The model under review builds one solid part; all positions refer to its coordinate system, in mm. A direction names the side the tool comes from. Coordinates: 2 decimals unless noted, no trailing zeros. Loops run counter-clockwise (first coordinate to the right, second up) from the corner with the lowest first, then second, coordinate; pieces in that order, holes last. Notation, with made-up numbers: M 61.5,2 L 71.5,2 A20 cw 71.5,41 Z; hole C -38.5,59.25 d2. An arc over 180 degrees is marked long. Write item = value, one per line. Start each with the question number.
Q1. Clearance check with flat-ended pins moving along their axes: pin 1 Ø1.5 at (x, y) = (6.5, 7.5) entering from -Z; pin 2 Ø1 at (x, z) = (4, 5) entering from -Y; pin 3 Ø2 at (y, z) = (9.5, -3) entering from +X. State where each tip first meets the part, or that it passes through.
Q2. We need section B-B on y = 4.25. Give the boundary of the cut face in (x, z), and give its area (3 significant figures).
Q3. For faces 1 (the face through (-4, 14.5, -6)), 2 (the face through (6.7, 8, -6.7)), 3 (the face through (-9.2, 0, 0.8)), list the 3-axis set-ups (+Z, -Z, +X, -X, +Y, -Y) from which the entire face can be reached by the end or side of a thin tool; tool diameter is ignored.
Q4. Mouldability with a two-part tool opening along X and no side actions: class faces 4 (the face through (0, 8, -10)), 5 (the face through (9.2, 0, 0.8)), 6 (the face through (-5.158, 14.732, 3.955)) as released by +X, released by -X, zero draft, split by the parting line, or undercut.
Q5. Wall thickness on probe 1 along Z at (x, y) = (0, 14.8); probe 2 along X at (y, z) = (15.4, 0); probe 3 along X at (y, z) = (4.5, 0): over which ranges is each line inside the solid? List them lowest first.
Q6. We need section A-A on z = 0. Give the boundary of the cut face in (x, y), and give its area (3 significant figures).
Q7. We need section D-D on y = 14. Give the boundary of the cut face in (x, z).
Q8. We need section C-C on x = 0. Give the boundary of the cut face in (y, z), and give its area (3 significant figures).
from build123d import *

# Parameters (mm, degrees)
F3_DEPTH = 8
F5_DEPTH = 16.001


with BuildPart() as f1:
    # F0 (on Top) → F1 (revolve)
    with BuildSketch(Plane.XY):
        Polygon((9, 0), (10, 0), (10, 16), (8, 16), (8, 14.5), (7, 14.5), (7, 16), (6.5, 16), (6.5, 13.5), (6, 13.5), (9, 9.9451635033), align=None)
    revolve(axis=Axis((0, 8.0098584294, 0), (0, 1, 0)))

    # F2 (on face) → F3 (cut)
    with BuildSketch(Plane.XZ):
        with BuildLine():
            Line((-6.8920810625, -7.2456344531), (-6.1847286297, -6.5382820203))
            ThreePointArc((-6.1847286297, -6.5382820203), (-6.3639610307, -6.3639610307), (-6.5382820203, -6.1847286297))
            Line((-6.5382820203, -6.1847286297), (-7.2456344531, -6.8920810625))
            ThreePointArc((-7.2456344531, -6.8920810625), (-7.0710678119, -7.0710678119), (-6.8920810625, -7.2456344531))
        make_face()
        with BuildLine():
            Line((7.2454194103, -6.8923071296), (6.5380675904, -6.1849553097))
            ThreePointArc((6.5380675904, -6.1849553097), (6.3639610307, -6.3639610307), (6.1849553097, -6.5380675904))
            Line((6.1849553097, -6.5380675904), (6.8923071296, -7.2454194103))
            ThreePointArc((6.8923071296, -7.2454194103), (7.0710678119, -7.0710678119), (7.2454194103, -6.8923071296))
        make_face()
    extrude(amount=-F3_DEPTH, mode=Mode.SUBTRACT)

    # F4 (on face) → F5 (cut, through all)
    with BuildSketch(Plane.XZ):
        with BuildLine():
            Line((-4.9749371855, 7.5), (0, 7.5))
            Line((0, 7.5), (4.9749371855, 7.5))
            ThreePointArc((4.9749371855, 7.5), (0, 9), (-4.9749371855, 7.5))
        make_face()
        with BuildLine():
            ThreePointArc((-4.9749371855, 7.5), (0, 9), (4.9749371855, 7.5))
            Line((4.9749371855, 7.5), (6.6143782777, 7.5))
            ThreePointArc((6.6143782777, 7.5), (0, 10), (-6.6143782777, 7.5))
            Line((-6.6143782777, 7.5), (-4.9749371855, 7.5))
        make_face()
    extrude(amount=-F5_DEPTH, mode=Mode.SUBTRACT)


solid = f1.part
Returned:
q1.pin_1 = -8.18
q1.pin_2 = 12.43
q1.pin_3 = 9.8
q2.outline = M -7.25,-6.89 L -6.54,-6.18 A9 cw -4.97,7.5 L -6.61,7.5 A10 ccw Z; M -6.89,-7.25 A10 ccw 6.89,-7.25 L 6.18,-6.54 A9 cw -6.18,-6.54 Z; M 4.97,7.5 A9 cw 6.54,-6.18 L 7.25,-6.89 A10 ccw 6.61,7.5 Z
q2.area = 46.2 mm^2
q3.face_1 = +Y
q3.face_2 = -Y
q3.face_3 = +Z, -Z, +X, -X, -Y
q4.face_4 = split by the parting line
q4.face_5 = zero draft
q4.face_6 = undercut
q5.probe_1 = -10 to -8, -7 to -6.5, 6.5 to 7
q5.probe_2 = -10 to -8, -7 to -6.5, 6.5 to 7, 8 to 10
q5.probe_3 = -10 to -9, 9 to 10
q6.outline = M -10,0 L -9,0 L -9,9.95 L -6,13.5 L -6.5,13.5 L -6.5,16 L -7,16 L -7,14.5 L -8,14.5 L -8,16 L -10,16 Z; M 6,13.5 L 9,9.95 L 9,0 L 10,0 L 10,16 L 8,16 L 8,14.5 L 7,14.5 L 7,16 L 6.5,16 L 6.5,13.5 Z
q6.area = 52.2 mm^2
q7.outline = M -6.61,7.5 A10 ccw long 6.61,7.5 Z; hole C 0,0 d13
q8.outline = M 0,-10 L 16,-10 L 16,-8 L 14.5,-8 L 14.5,-7 L 16,-7 L 16,-6.5 L 13.5,-6.5 L 13.5,-6 L 9.95,-9 L 0,-9 Z; M 11.72,7.5 L 13.5,6 L 13.5,6.5 L 16,6.5 L 16,7 L 14.5,7 L 14.5,7.5 Z
q8.area = 29.2 mm^2
